Build history of the part. All positions in model axes, mm. A direction names the side the tool comes from. Give positions to 0.01 mm unless a question says otherwise; leave off trailing zeros. Write each loop counter-clockwise with the first axis right and the second up, starting at its lowest first coordinate (ties: lowest second). Pieces come first, ordered by that corner, then holes. Notation, with made-up numbers: M -26,18.5 L 3,18.5 A15 ccw 3,32.5 Z; hole C -4.5,43 d6. An arc over 180 degrees is marked long. Return JSON: item names as keys, results as strings. Group by question number.
Q1. Band-saw the part on A-A, the plane y = 12.7. Give the cut face in (x, z).
Q2. Pull direction Y, two halves, no side cores. Call faces 6 (the flat face through (53, 19.05, 0)), 7 (the flat face through (55.88, 13, 0)), 8 (the flat face through (-1, 0, 0)): +Y half, -Y half, draft (parallel to the pull), parting line (faces both ways), or undercut.
Q3. Wall check: probe 1 along Z at (x, y) = (26, 22.5); probe 2 along X at (y, z) = (12.5, 38.5); probe 3 along X at (y, z) = (21, 5.5). Give the ranges that are in metal, low to high.
Q4. Band-saw the part on B-B, the plane z = 8.5. Give the cut face in (x, y).
Q5. Band-saw the part on C-C, the plane x = 37.5. Give the cut face in (y, z), then the cut area to 3 significant figures.
Q6. Flat gauge pins, fed straight in: pin 1 Ø5 at (x, y) = (39, 19.5) entering from +Z; pin 2 Ø5.5 at (x, y) = (54.5, 15) entering from +Z; pin 3 Ø1.5 at (x, z) = (53, -3) entering from -Y. Where does each tip first touch, or does it go through?
Q7. Band-saw the part on D-D, the plane z = 35. Give the cut face in (x, y), then the cut area to 3 significant figures.
Q8. Tool access for faces 1 (the flat face through (53, 13, -6.35)), 2 (the cylindrical face through (-2.43, 15.22, 31.48)), 3 (the flat face through (53, 13, 6.35)), 4 (the flat face through (53, 6.35, 0)), 5 (the flat face through (-50.8, 13, 0)): list every direction of +Z, -Z, +X, -X, +Y, -Y with a clear straight run to the whole face (end or side of a thin tool).
from build123d import *

# Parameters (mm, degrees)
SKETCH1_W           = 101.6
SKETCH1_H           = 25.4
BOSS_EXTRUDE1_DEPTH = 25.4
SKETCH2_W           = 12.7
SKETCH2_H           = 12.7
BOSS_EXTRUDE2_DEPTH = 5.08
SKETCH6_R           = 2.54
BOSS_EXTRUDE4_DEPTH = 38.1


with BuildPart() as part:
    # Sketch1 → Boss-Extrude1 (new body)
    with BuildSketch(Plane(origin=(0, 0, 0), x_dir=(1, 0, 0), z_dir=(0, 1, 0))):
        Rectangle(SKETCH1_W, SKETCH1_H)
    extrude(amount=BOSS_EXTRUDE1_DEPTH)

    # Sketch2 → Boss-Extrude2 (add)
    with BuildSketch(Plane(origin=(50.8, 0, 0), x_dir=(0, 0, -1), z_dir=(1, 0, 0))):
        with Locations((0, 12.7)):
            Rectangle(SKETCH2_W, SKETCH2_H)
    extrude(amount=BOSS_EXTRUDE2_DEPTH)

    # Sketch6 → Boss-Extrude4 (add)
    with BuildSketch(Plane.XY.offset(12.7)):
        with Locations((-2.101074924, 12.7)):
            Circle(SKETCH6_R)
    extrude(amount=BOSS_EXTRUDE4_DEPTH)


solid = part.part
From the geometry:
{
 "1": {"outline": "M -50.8,-12.7 L 50.8,-12.7 L 50.8,-6.35 L 55.88,-6.35 L 55.88,6.35 L 50.8,6.35 L 50.8,12.7 L 0.44,12.7 L 0.44,50.8 L -4.64,50.8 L -4.64,12.7 L -50.8,12.7 Z"},
 "2": {"face 6": "+Y half", "face 7": "draft", "face 8": "-Y half"},
 "3": {"probe 1": "z = -12.7 to 12.7", "probe 2": "x = -4.63 to 0.43", "probe 3": "x = -50.8 to 50.8"},
 "4": {"outline": "M -50.8,0 L 50.8,0 L 50.8,25.4 L -50.8,25.4 Z"},
 "5": {"outline": "M 0,-12.7 L 25.4,-12.7 L 25.4,12.7 L 0,12.7 Z", "area": "645 mm^2"},
 "6": {"pin 1": "stops at z = 12.7", "pin 2": "stops at z = 6.35", "pin 3": "stops at y = 6.35"},
 "7": {"outline": "C -2.1,12.7 d5.08", "area": "20.3 mm^2"},
 "8": {"face 1": "-Z, +X, +Y, -Y", "face 2": "+Z", "face 3": "+Z, +X, +Y, -Y", "face 4": "+Z, -Z, +X, -Y", "face 5": "+Z, -Z, -X, +Y, -Y"}
}
